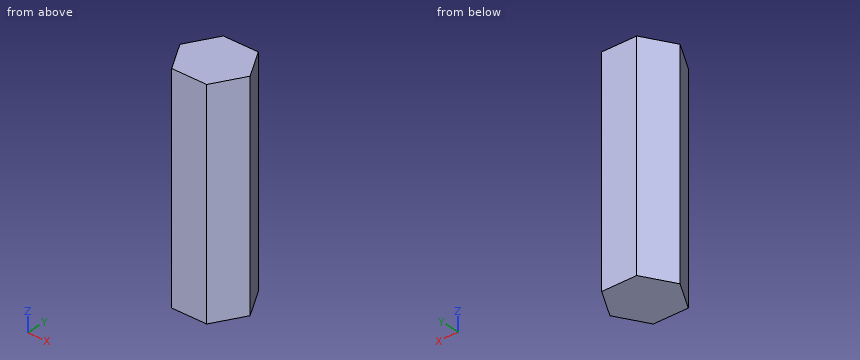
from build123d import *

# Parameters (mm, degrees)
F1_DEPTH = 254
F2_R     = 23.522227
F3_DEPTH = 111.76


with BuildPart() as f1:
    # F0 (on Top) → F1 (new body)
    with BuildSketch(Plane.XY):
        Polygon((-21.18477, 35.333617), (-41.192195, -0.679741), (-20.007425, -36.013357), (21.18477, -35.333617), (41.192195, 0.679741), (20.007425, 36.013357), align=None)
    extrude(amount=F1_DEPTH)

    # F2 (on face) → F3 (join)
    with BuildSketch(Plane.XY.offset(254)):
        Circle(F2_R)
    extrude(amount=-F3_DEPTH)


solid = f1.part
Can you work these out from the model? Positions are in its coordinate system, mm. Give positions to 0.01 mm unless a question says otherwise; leave off trailing zeros. Loops run counter-clockwise (first coordinate to the right, second up) from the corner with the lowest first, then second, coordinate; pieces in that order, holes last. Notation, with made-up numbers: (5, 67.5) - (19, 67.5) arc R32 cw to (19, 105.5) - close; hole circle Ø7 at (47, -2.5). An arc over 180 degrees is marked (long way). One line per item, written item: value.
(1) I need wall thicknesses on line 1 along Y through (x, z) = (20, 126); line 2 along X through (y, z) = (23, 175); line 3 along Y through (x, z) = (-27.5, 203.5). Which ranges of each line are inside material? Lowest first, please.
Verdict:
line 1: -35.35 to 36.01
line 2: -28.04 to 27.81
line 3: -23.52 to 23.97
(2) If we section it at A-A, the plane z = 73.5: List the corners of the cut face in (x, y) for me.
Verdict:
outline: (-41.19, -0.68) - (-20.01, -36.01) - (21.18, -35.33) - (41.19, 0.68) - (20.01, 36.01) - (-21.18, 35.33) - close
(3) If we section it at B-B, the plane y = -27.5: List the corners of the cut face in (x, z) for me.
Verdict:
outline: (-25.11, 0) - (25.54, 0) - (25.54, 254) - (-25.11, 254) - close
(4) If we section it at C-C, the plane x = 27.5: List the corners of the cut face in (y, z) for me.
Verdict:
outline: (-23.97, 0) - (23.52, 0) - (23.52, 254) - (-23.97, 254) - close
(5) I'm going to push flat-ended pins straight in: pin 1 (10 mm diameter, centred on y = -21.5, z = 146, fed in from -X); pin 2 (8 mm diameter, centred on x = -31, y = 15, fed in from -Z); pin 3 (10 mm diameter, centred on y = 15, z = 137, fed in from -X). Where does each tip first touch, or does it pass through?
Verdict:
pin 1: x = -31.71
pin 2: z = 0
pin 3: x = -35.26
